from build123d import *

# Parameters (mm, degrees)
F1_DEPTH = 3.175


with BuildPart() as f1:
    # F0 (on Top) → F1 (new body)
    with BuildSketch(Plane.XY):
        Polygon((53.419934, 62.122178), (-52.802866, 62.122178), (-52.802866, 57.49908), (-52.802866, 48.79114), (-52.802866, 7.30868), (-52.802866, -1.39926), (-52.802866, -16.135222), (53.419934, -16.135222), align=None)
        Polygon((-52.802866, 7.30868), (-52.802866, 48.79114), (-73.326066, 48.79114), (-73.326066, -1.39926), (-52.802866, -1.39926), align=None)
    extrude(amount=F1_DEPTH)


solid = f1.part
Build history of the part. All positions in model axes, mm. A direction names the side the tool comes from. Round coordinates to 2 decimals unless told otherwise and drop trailing zeros. Loops run counter-clockwise (first coordinate to the right, second up) from the corner with the lowest first, then second, coordinate; pieces in that order, holes last. Notation, with made-up numbers: (47, 31.25) -> (81, 31.25) arc R16 ccw to (81, 43.25) -> close; hole circle Ø11 at (45, 13.25). An arc over 180 degrees is marked (long way). One line per item, written item: value. Start each with the question number.
Q1. Two-plate mould, pull along Y, no slides. Class faces 4 (the face through (-63, -1.399, 2)), 5 (the face through (1, 62.122, 2)), 6 (the face through (-73.326, 24, 2)): released by +Y, released by -Y, zero draft, split by the parting line, or undercut.
Q2. Cut at B-B on x = -62.5. List the corners of the cut face in (y, z) (3 decimals), plus the area to 3 significant figures.
Q3. 3-axis set-ups, long thin cutter, end or side, ignore diameter. For faces 1 (the face through (-63, 48.791, 2)), 2 (the face through (-52.803, -9, 2)), 3 (the face through (0, -16.135, 2)): which of +Z, -Z, +X, -X, +Y, -Y reach the whole face in a straight line?
Q4. Cut at A-A on z = 2.6. List the corners of the cut face in (x, y), plus the area to 3 significant figures.
Q5. Probe line 1 along X through (y, z) = (59, 2.5); line 2 along Y through (x, z) = (-62.5, 3.05). List the from-to ranges inside material, lowest first.
Q6. Drop flat-ended pins along their axis: pin 1 Ø1 at (x, z) = (-63.5, 1) entering from -Y; pin 2 Ø1 at (y, z) = (58.5, 1.5) entering from -X. Give the stop position or say it passes through.
Computed:
1. face 4: released by -Y
1. face 5: released by +Y
1. face 6: zero draft
2. outline: (-1.399, 0) -> (48.791, 0) -> (48.791, 3.175) -> (-1.399, 3.175) -> close
2. area: 159 mm²
3. face 1: +Z, -Z, -X, +Y
3. face 2: +Z, -Z, -X, -Y
3. face 3: +Z, -Z, +X, -X, -Y
4. outline: (-73.33, -1.4) -> (-52.8, -1.4) -> (-52.8, -16.14) -> (53.42, -16.14) -> (53.42, 62.12) -> (-52.8, 62.12) -> (-52.8, 48.79) -> (-73.33, 48.79) -> close
4. area: 9,340 mm²
5. line 1: -52.8 to 53.42
5. line 2: -1.4 to 48.79
6. pin 1: y = -1.4
6. pin 2: x = -52.8
